Build history of the part. All positions in model axes, mm. Face numbers are marked on the shaded views. Round coordinates to 2 decimals unless told otherwise and drop trailing zeros. Write each loop counter-clockwise with the first axis right and the second up, starting at its lowest first coordinate (ties: lowest second). Pieces come first, ordered by that corner, then holes.
from build123d import *

# Parameters (mm, degrees)
F0_W     = 50.8
F0_H     = 50.8
F1_DEPTH = 25.4
F2_R     = 12.7
F3_DEPTH = 25.4
F4_R     = 5.08


with BuildPart() as f1:
    # F0 (on Top) → F1 (new body)
    with BuildSketch(Plane.XY):
        with Locations((2.406318, -0.585664)):
            Rectangle(F0_W, F0_H)
    extrude(amount=F1_DEPTH)

    # F2 (on face) → F3 (cut)
    with BuildSketch(Plane.XY.offset(25.4)):
        Circle(F2_R)
    extrude(amount=-F3_DEPTH, mode=Mode.SUBTRACT)

    # F4
    f4_edges = [f1.edges().sort_by_distance(p)[0] for p in [
        (2.406318, -25.985664, 25.4),
        (27.806318, -0.585664, 25.4),
        (2.406318, 24.814336, 25.4),
        (-22.993682, -0.585664, 25.4),
    ]]
    fillet(f4_edges, radius=F4_R)


solid = f1.part
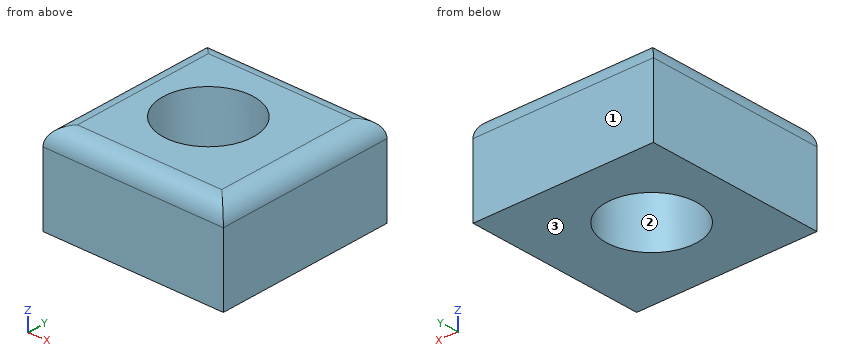
1) Slice it at B-B (z = 5.5). Write the cut outline in (x, y), plus the area to 3 significant figures.
Results:
outline: (-22.99, -25.99) - (27.81, -25.99) - (27.81, 24.81) - (-22.99, 24.81) - close; hole circle Ø25.4 at (0, 0)
area: 2,070 mm2
2) Mould opens along Y. For the marked faces 1, 2 and 3 say: released by +Y, released by -Y, zero draft, split by the parting line, or undercut.
Results:
face 1: released by +Y
face 2: undercut
face 3: zero draft
3) Wall check: L1, parallel to Y at x = 0, z = 7.25; L2, parallel to X at y = 0.5, z = 18.5; L3, parallel to Y at x = -6, z = 11.25. Give the ranges that are in metal, low to high.
Results:
L1: y = -25.99 to -12.7, 12.7 to 24.81
L2: x = -22.99 to -12.69, 12.69 to 27.81
L3: y = -25.99 to -11.19, 11.19 to 24.81
4) Slice it at A-A (y = 0). Write the cut outline in (x, z), plus the area to 3 significant figures.
Results:
outline: (-22.99, 0) - (-12.7, 0) - (-12.7, 25.4) - (-17.91, 25.4) arc R5.08 ccw to (-22.99, 20.32) - close; (12.7, 0) - (27.81, 0) - (27.81, 20.32) arc R5.08 ccw to (22.73, 25.4) - (12.7, 25.4) - close
area: 634 mm2
5) Pin check, flat tip, straight feed: pin 1 Ø12 at (x, y) = (-9.5, 6.5) entering from -Z. Stop position of the tip, or through.
Results:
pin 1: stops at z = 0
6) Slice it at D-D (z = 21.25). Write the cut outline in (x, y), plus the area to 3 significant figures.
Results:
outline: (-22.91, -25.9) - (27.72, -25.9) - (27.72, 24.73) - (-22.91, 24.73) - close; hole circle Ø25.4 at (0, 0)
area: 2,060 mm2
7) Slice it at C-C (x = 0). Write the cut outline in (y, z), plus the area to 3 significant figures.
Results:
outline: (-25.99, 0) - (-12.7, 0) - (-12.7, 25.4) - (-20.91, 25.4) arc R5.08 ccw to (-25.99, 20.32) - close; (12.7, 0) - (24.81, 0) - (24.81, 20.32) arc R5.08 ccw to (19.73, 25.4) - (12.7, 25.4) - close
area: 634 mm2
